CAD build for the part. Positions are in the model's coordinates, mm. Round coordinates to 2 decimals unless told otherwise and drop trailing zeros. Loops run counter-clockwise (first coordinate to the right, second up) from the corner with the lowest first, then second, coordinate; pieces in that order, holes last. Notation, with made-up numbers: (47, 34.25) -> (100, 34.25) arc R22 ccw to (100, 61.25) -> close; hole circle Ø2 at (62.5, 55). An arc over 180 degrees is marked (long way). Answer as CSV lines item,"result".
```python
from build123d import *

# Parameters (mm, degrees)
F1_DEPTH = 50.8


with BuildPart() as f1:
    # F0 (on Front) → F1 (new body)
    with BuildSketch(Plane.XZ):
        Polygon((0, 50.8), (0, 0), (50.8, 0), (50.8, 2.1089113951), (50.8, 50.8), align=None)
    extrude(amount=F1_DEPTH)

    # F2 (on face) → F3 (revolve, cut)
    with BuildSketch(Plane.YZ.offset(50.8)):
        with BuildLine():
            ThreePointArc((-31.75, 38.1), (-35.6699602045, 43.9666350314), (-42.5901280605, 42.5901280605))
            Line((-42.5901280605, 42.5901280605), (-33.6098719395, 33.6098719395))
            ThreePointArc((-33.6098719395, 33.6098719395), (-32.2333649686, 35.6699602045), (-31.75, 38.1))
        make_face()
        with BuildLine():
            ThreePointArc((-6.35, 12.7), (-10.2699602045, 18.5666350314), (-17.1901280605, 17.1901280605))
            Line((-17.1901280605, 17.1901280605), (-8.2098719395, 8.2098719395))
            ThreePointArc((-8.2098719395, 8.2098719395), (-6.8333649686, 10.2699602045), (-6.35, 12.7))
        make_face()
    revolve(axis=Axis((50.8, -25.4, 25.4), (0, 0.7071067812, -0.7071067812)), mode=Mode.SUBTRACT)

    # F4 (on face) → F5 (revolve, cut)
    with BuildSketch(Plane.XZ.offset(50.8)):
        with BuildLine():
            Line((25.4, 19.05), (25.4, 31.75))
            ThreePointArc((25.4, 31.75), (19.05, 25.4), (25.4, 19.05))
        make_face()
    revolve(axis=Axis((25.4, -50.8, 25.4), (0, 0, -1)), mode=Mode.SUBTRACT)

    # F6 (on face) → F7 (revolve, cut)
    with BuildSketch(Plane(origin=(0, 0, 0), x_dir=(-1, 0, 0), z_dir=(0, 1, 0))):
        with BuildLine():
            Line((-17.1901280605, 17.1901280605), (-8.2098719395, 8.2098719395))
            ThreePointArc((-8.2098719395, 8.2098719395), (-6.8333649686, 10.2699602045), (-6.35, 12.7))
            ThreePointArc((-6.35, 12.7), (-10.2699602045, 18.5666350314), (-17.1901280605, 17.1901280605))
        make_face()
        with BuildLine():
            ThreePointArc((-19.05, 25.4), (-22.9699602045, 31.2666350314), (-29.8901280605, 29.8901280605))
            Line((-29.8901280605, 29.8901280605), (-20.9098719395, 20.9098719395))
            ThreePointArc((-20.9098719395, 20.9098719395), (-19.5333649686, 22.9699602045), (-19.05, 25.4))
        make_face()
        with BuildLine():
            ThreePointArc((-31.75, 38.1), (-35.6699602045, 43.9666350314), (-42.5901280605, 42.5901280605))
            Line((-42.5901280605, 42.5901280605), (-33.6098719395, 33.6098719395))
            ThreePointArc((-33.6098719395, 33.6098719395), (-32.2333649686, 35.6699602045), (-31.75, 38.1))
        make_face()
    revolve(axis=Axis((25.4, 0, 25.4), (-0.7071067812, 0, -0.7071067812)), mode=Mode.SUBTRACT)


solid = f1.part
```
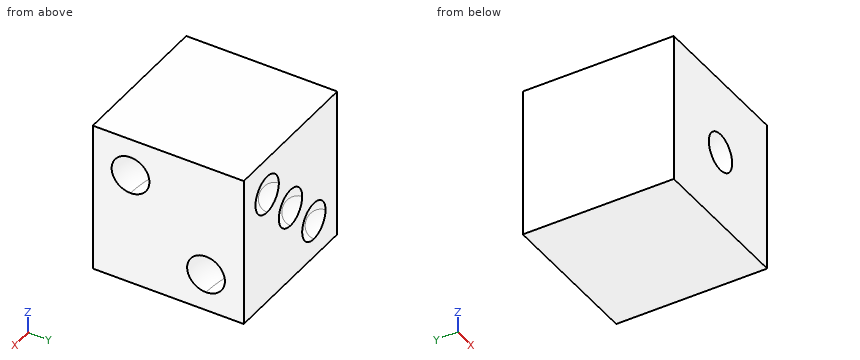
Q1. Slice it at C-C, the plane z = 24. Give the cut face in (x, y).
Results:
outline,"(0, -50.8) -> (19.21, -50.8) arc R6.19 cw to (31.59, -50.8) -> (50.8, -50.8) -> (50.8, 0) -> (31.59, 0) arc R6.19 cw to (19.21, 0) -> (0, 0) -> close"
Q2. Probe L1, parallel to Z at x = 48, y = -38; L2, parallel to Z at x = 27.5, y = -48; L3, parallel to Y at x = 28, z = 25. List the from-to ranges inside material, lowest first. Write a range as [from, to].
Results:
L1,"[0, 32.4], [43.8, 50.8]"
L2,"[0, 20.1], [30.7, 50.8]"
L3,"[-45.02, -5.78]"
Q3. Slice it at A-A, the plane y = -9. Give the cut face in (x, z), and give its area (3 significant figures).
Results:
outline,"(0, 0) -> (50.8, 0) -> (50.8, 7.54) arc R5.16 cw to (50.8, 17.86) -> (50.8, 50.8) -> (0, 50.8) -> close"
area,"2,540 mm2"
Q4. Slice it at B-B, the plane x = 23.5. Give the cut face in (y, z).
Results:
outline,"(-50.8, 0) -> (0, 0) -> (0, 19.34) arc R6.06 cw to (0, 31.46) -> (0, 50.8) -> (-50.8, 50.8) -> (-50.8, 31.46) arc R6.06 cw to (-50.8, 19.34) -> close"
Q5. Slice it at D-D, the plane y = -46. Give the cut face in (x, z).
Results:
outline,"(0, 0) -> (50.8, 0) -> (50.8, 50.8) -> (0, 50.8) -> close; hole circle Ø8.31 at (25.4, 25.4)"
